from build123d import *

# Parameters (mm, degrees)
SKETCH1_W           = 40
SKETCH1_H           = 45
BOSS_EXTRUDE1_DEPTH = 70
SKETCH2_R           = 12.5
CUT_EXTRUDE1_DEPTH  = 10
SKETCH3_R           = 12.5
CUT_EXTRUDE2_DEPTH  = 10
SKETCH4_W           = 40
SKETCH4_H           = 22.5
CUT_EXTRUDE3_DEPTH  = 71
SKETCH5_W           = 40
SKETCH5_H           = 50
CUT_EXTRUDE4_DEPTH  = 15


with BuildPart() as part:
    # Sketch1 → Boss-Extrude1 (new body)
    with BuildSketch(Plane.XY):
        Rectangle(SKETCH1_W, SKETCH1_H)
    extrude(amount=BOSS_EXTRUDE1_DEPTH)

    # Sketch2 → Cut-Extrude1 (cut)
    with BuildSketch(Plane(origin=(0, 0, 0), x_dir=(-1, 0, 0), z_dir=(0, 0, -1))):
        Circle(SKETCH2_R)
    extrude(amount=-CUT_EXTRUDE1_DEPTH, mode=Mode.SUBTRACT)

    # Sketch3 → Cut-Extrude2 (cut)
    with BuildSketch(Plane.XY.offset(70)):
        Circle(SKETCH3_R)
    extrude(amount=-CUT_EXTRUDE2_DEPTH, mode=Mode.SUBTRACT)

    # Sketch4 → Cut-Extrude3 (cut, through all)
    with BuildSketch(Plane.XY.offset(70)):
        with Locations((0, 11.25)):
            Rectangle(SKETCH4_W, SKETCH4_H)
    extrude(amount=-CUT_EXTRUDE3_DEPTH, mode=Mode.SUBTRACT)

    # Sketch5 → Cut-Extrude4 (cut)
    with BuildSketch(Plane(origin=(0, 0, 0), x_dir=(1, 0, 0), z_dir=(0, 1, 0))):
        with Locations((0, -35)):
            Rectangle(SKETCH5_W, SKETCH5_H)
    extrude(amount=-CUT_EXTRUDE4_DEPTH, mode=Mode.SUBTRACT)


solid = part.part
The listing builds one solid part. Answer for the finished solid, in the listing's coordinates (mm). A direction names the side the tool comes from. Round coordinates to 2 decimals unless told otherwise and drop trailing zeros. Order: outer loops, then holes, each group sorted by start corner. A loop starts at its lowest first (then second) coordinate and runs counter-clockwise, first axis right, second up. Notation, with made-up numbers: (-12, -8) - (46, -8) arc R11 ccw to (46, -4) - close; hole circle Ø7 at (-32, -26.75). An arc over 180 degrees is marked (long way). Write item = value, one per line. Start each with the question number.
1) Section C-C, the plane z = 63 is taken. Write down the section's boundary in (x, y), plus the area to 3 significant figures.
2) Section A-A, the plane x = 13.5 is taken. Write down the section's boundary in (y, z).
3) Section B-B, the plane y = -11.5 is taken. Write down the section's boundary in (x, z).
4) Section D-D, the plane x = 0 is taken. Write down the section's boundary in (y, z), plus the area to 3 significant figures.
5) Straight lines are drawn through the part: L1, parallel to Z at x = 12.5, y = -6.25; L2, parallel to Y at x = 18, z = 40; L3, parallel to X at y = -9.5, z = 61. For each, find the intervals that lie inside material, in ascending order.
6) Given pin 1 (6 mm diameter, centred on x = -12.5, z = 16, fed in from +Y); pin 2 (12 mm diameter, centred on x = -2, y = -5, fed in from -Z), each flat-ended and moving along its own axis, determine where each tip first touches the part or whether it passes through.
7) For faces 5 (the flat face through (0, -14, 10)), 6 (the flat face through (0, -14, 0)), determine the directions among +Z, -Z, +X, -X, +Y, -Y from which every point of the face is accessible in a straight line to the end or side of a thin tool.
8) For a pull along X with two mould halves and no side action, classify faces 1 (the flat face through (-20, -16, 35)), 2 (the flat face through (20, -16, 35)), 3 (the cylindrical face through (0.275, -12.497, 4.93)), 4 (the flat face through (-16, 0, 5)) as released by +X, released by -X, zero draft, split by the parting line, or undercut.
Results list:
q1.outline = (-20, -22.5) - (20, -22.5) - (20, 0) - (12.5, 0) arc R12.5 cw to (-12.5, 0) - (-20, 0) - close
q1.area = 655 mm^2
q2.outline = (-22.5, 0) - (0, 0) - (0, 10) - (-15, 10) - (-15, 60) - (0, 60) - (0, 70) - (-22.5, 70) - close
q3.outline = (-20, 0) - (-4.9, 0) - (-4.9, 10) - (-20, 10) - close; (-20, 60) - (-4.9, 60) - (-4.9, 70) - (-20, 70) - close; (4.9, 0) - (20, 0) - (20, 10) - (4.9, 10) - close; (4.9, 60) - (20, 60) - (20, 70) - (4.9, 70) - close
q4.outline = (-22.5, 0) - (-12.5, 0) - (-12.5, 10) - (-15, 10) - (-15, 60) - (-12.5, 60) - (-12.5, 70) - (-22.5, 70) - close
q4.area = 575 mm^2
q5.L1 = 0 to 10, 60 to 70
q5.L2 = -22.5 to -15
q5.L3 = -20 to -8.12, 8.12 to 20
q6.pin_1 = -15
q6.pin_2 = through
q7.face_5 = +X, -X, +Y
q7.face_6 = -Z, +X, -X, +Y, -Y
q8.face_1 = released by -X
q8.face_2 = released by +X
q8.face_3 = undercut
q8.face_4 = zero draft
